Geometry check sheet. Reference: the model listing, model coordinates, mm. Round coordinates to 2 decimals unless told otherwise and drop trailing zeros. Order: outer loops, then holes, each group sorted by start corner. A loop starts at its lowest first (then second) coordinate and runs counter-clockwise, first axis right, second up. Notation, with made-up numbers: (28.5, 82) - (43.5, 82) arc R20 ccw to (43.5, 108) - close; hole circle Ø3 at (-2, 83). An arc over 180 degrees is marked (long way). Use a Markdown table: item, result. Add a question column.
(1) Section check A-A on x = 44. Record the boundary of the cut face in (y, z) (3 decimals), then the cut area to 4 significant figures.
(2) Gauge pin test, flat ends, axial feed: P1, Ø1, axis at x = 144.5, z = -1.5, coming from the +Y side; P2, Ø1.6, axis at y = -14, z = -1, coming from the -X side. Record the tip position at first contact, or that the pin passes through.
(3) Thickness scan on line 1 along X through (y, z) = (-157, -0.8); line 2 along X through (y, z) = (-180.6, -0.9); line 3 along Y through (x, z) = (216, -2.5). Record the ranges inside material, lowest first. Write a range as [from, to].
(4) Section check C-C on x = 115. Record the boundary of the cut face in (y, z) (3 decimals).
(5) Section check B-B on z = -0.55. Give the number of separate pieces and of enclosed holes in the cut face, then the cut area to 3 significant figures.
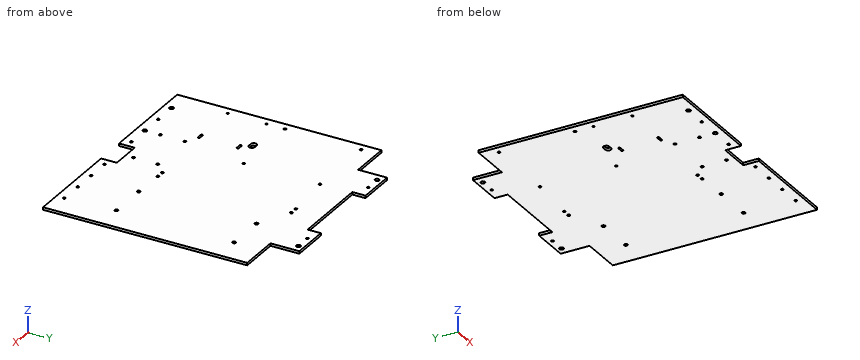
```python
from build123d import *

# Parameters (mm, degrees)
SKETCH1_W                    = 300
SKETCH1_H                    = 300
BOSS_EXTRUDE1_DEPTH          = 3.175
SKETCH2_W                    = 52
SKETCH2_H                    = 40
CUT_EXTRUDE1_DEPTH           = 10
M4_START                     = -3.175
M4_CLEARANCE_HOLE1_OUTLINE_R = 2.15
M4_CLEARANCE_HOLE1_DEPTH     = 3.175
M3_CLEARANCE_HOLE2_D         = 3.2
M2_5_CLEARANCE_HOLE1_D       = 2.7
M3_CLEARANCE_HOLE3_D         = 3.2
M3_CLEARANCE_HOLE4_D         = 3.2
CUT_EXTRUDE3_DEPTH           = 10
CUT_EXTRUDE4_DEPTH           = 10
SKETCH15_W                   = 40
SKETCH15_H                   = 20
CUT_EXTRUDE5_DEPTH           = 10
CUT_EXTRUDE6_START           = -10
CUT_EXTRUDE6_DEPTH           = 10
M3_CLEARANCE_HOLE5_D         = 3.4
M5_CLEARANCE_HOLE1_D         = 5.5
M3_CLEARANCE_HOLE7_D         = 3.4


# Read off the part's stored shape, not the designer's step: M4 Clearance Hole1
with BuildPart() as part:
    # Sketch1 → Boss-Extrude1 (new body)
    with BuildSketch(Plane(origin=(0, 0, 0), x_dir=(1, 0, 0), z_dir=(0, 0, -1))):
        with Locations((150, 150)):
            Rectangle(SKETCH1_W, SKETCH1_H)
    extrude(amount=BOSS_EXTRUDE1_DEPTH)

    # Sketch2 → Cut-Extrude1 (cut)
    with BuildSketch(Plane(origin=(0, 0, -3.175), x_dir=(1, 0, 0), z_dir=(0, 0, -1))):
        with Locations((26, 20)):
            Rectangle(SKETCH2_W, SKETCH2_H)
        with Locations((274, 20)):
            Rectangle(SKETCH2_W, SKETCH2_H)
    extrude(amount=-CUT_EXTRUDE1_DEPTH, mode=Mode.SUBTRACT)

    # M4 Clearance Hole1 outline → M4 Clearance Hole1 (cut)
    with BuildSketch(Plane.XY.offset(M4_START)):
        with Locations((266, -226)):
            Circle(M4_CLEARANCE_HOLE1_OUTLINE_R)
        with Locations((216, -76)):
            Circle(M4_CLEARANCE_HOLE1_OUTLINE_R)
        with Locations((216, -226)):
            Circle(M4_CLEARANCE_HOLE1_OUTLINE_R)
        with Locations((266, -76)):
            Circle(M4_CLEARANCE_HOLE1_OUTLINE_R)
    extrude(amount=M4_CLEARANCE_HOLE1_DEPTH, mode=Mode.SUBTRACT)

    # M3 Clearance Hole2 (through all)
    with Locations(Plane(origin=(0, 0, -3.175), x_dir=(-1, 0, 0), z_dir=(0, 0, -1))):
        with Locations((-102, -60), (-10, -157), (-102, -157), (-10, -60)):
            Hole(M3_CLEARANCE_HOLE2_D / 2)

    # M2.5 Clearance Hole1 (through all)
    with Locations(Plane(origin=(0, 0, -3.175), x_dir=(-1, 0, 0), z_dir=(0, 0, -1))):
        with Locations((-74, -180.6), (-10, -230), (-74, -230), (-10, -180.6), (-68, -230), (-68, -180.6)):
            Hole(M2_5_CLEARANCE_HOLE1_D / 2)

    # M3 Clearance Hole3 (through all)
    with Locations(Plane(origin=(0, 0, -3.175), x_dir=(-1, 0, 0), z_dir=(0, 0, -1))):
        with Locations((-30, -290), (-270, -290), (-240, -290), (-210, -290), (-180, -290), (-150, -290), (-120, -290), (-90, -290), (-60, -290)):
            Hole(M3_CLEARANCE_HOLE3_D / 2)

    # M3 Clearance Hole4 (through all)
    with Locations(Plane(origin=(0, 0, -3.175), x_dir=(-1, 0, 0), z_dir=(0, 0, -1))):
        with Locations((-82, -10), (-238, -10), (-150, -10), (-62, -10), (-218, -10)):
            Hole(M3_CLEARANCE_HOLE4_D / 2)

    # Sketch5 → Cut-Extrude3 (cut)
    with BuildSketch(Plane(origin=(0, 0, -3.175), x_dir=(-1, 0, 0), z_dir=(0, 0, -1))):
        Polygon((-248, 0), (-52, 0), (-52, -3.2), (-100, -3.2), (-100, -20), (-200, -20), (-200, -3.2), (-248, -3.2), align=None)
    extrude(amount=-CUT_EXTRUDE3_DEPTH, mode=Mode.SUBTRACT)

    # Sketch14 → Cut-Extrude4 (cut)
    with BuildSketch(Plane(origin=(0, 0, -3.175), x_dir=(-1, 0, 0), z_dir=(0, 0, -1))):
        with BuildLine():
            Line((-63, -165.2), (-59, -165.2))
            ThreePointArc((-59, -165.2), (-55.2, -169), (-59, -172.8))
            Line((-59, -172.8), (-63, -172.8))
            ThreePointArc((-63, -172.8), (-66.8, -169), (-63, -165.2))
        make_face()
    extrude(amount=-CUT_EXTRUDE4_DEPTH, mode=Mode.SUBTRACT)

    # Sketch15 → Cut-Extrude5 (cut)
    with BuildSketch(Plane(origin=(0, 0, -3.175), x_dir=(-1, 0, 0), z_dir=(0, 0, -1))):
        with Locations((-150, -290)):
            Rectangle(SKETCH15_W, SKETCH15_H)
    extrude(amount=-CUT_EXTRUDE5_DEPTH, mode=Mode.SUBTRACT)

    # Sketch16 → Cut-Extrude6 (cut)
    with BuildSketch(Plane(origin=(0, 0, -3.175), x_dir=(-1, 0, 0), z_dir=(0, 0, -1)).offset(CUT_EXTRUDE6_START)):
        with BuildLine():
            Line((-74, -179.25), (-68, -179.25))
            ThreePointArc((-68, -179.25), (-66.65, -180.6), (-68, -181.95))
            Line((-68, -181.95), (-74, -181.95))
            ThreePointArc((-74, -181.95), (-75.35, -180.6), (-74, -179.25))
        make_face()
        with BuildLine():
            Line((-74, -228.65), (-68, -228.65))
            ThreePointArc((-68, -228.65), (-66.65, -230), (-68, -231.35))
            Line((-68, -231.35), (-74, -231.35))
            ThreePointArc((-74, -231.35), (-75.35, -230), (-74, -228.65))
        make_face()
    extrude(amount=CUT_EXTRUDE6_DEPTH, mode=Mode.SUBTRACT)

    # M3 Clearance Hole5 (through all)
    with Locations(Plane(origin=(0, 0, -3.175), x_dir=(-1, 0, 0), z_dir=(0, 0, -1))):
        with Locations((-175, -55), (-165, -225), (-175, -225), (-165, -55)):
            Hole(M3_CLEARANCE_HOLE5_D / 2)

    # M5 Clearance Hole1 (through all)
    with Locations(Plane(origin=(0, 0, -3.175), x_dir=(-1, 0, 0), z_dir=(0, 0, -1))):
        with Locations((-62, -10), (-90, -290), (-30, -290), (-238, -10)):
            Hole(M5_CLEARANCE_HOLE1_D / 2)

    # M3 Clearance Hole7 (through all)
    with Locations(Plane(origin=(0, 0, -3.175), x_dir=(-1, 0, 0), z_dir=(0, 0, -1))):
        with Locations((-150.5, -239), (-90, -270), (-150.5, -270), (-90, -239)):
            Hole(M3_CLEARANCE_HOLE7_D / 2)


solid = part.part
```
Check sheet entries:
| question | item | result |
|---|---|---|
| 1 | outline | (-300, -3.175) - (-40, -3.175) - (-40, 0) - (-300, 0) - close |
| 1 | area | 825.5 mm2 |
| 2 | P1 | stops at y = -20 |
| 2 | P2 | stops at x = 52 |
| 3 | line 1 | x = [0, 8.4], [11.6, 100.4], [103.6, 300] |
| 3 | line 2 | x = [0, 8.65], [11.35, 66.65], [75.35, 300] |
| 3 | line 3 | y = [-300, -228.15], [-223.85, -78.15], [-73.85, -3.2] |
| 4 | outline | (-300, -3.175) - (-20, -3.175) - (-20, 0) - (-300, 0) - close |
| 5 | separate pieces | 1 |
| 5 | enclosed holes | 33 |
| 5 | area | 82,300 mm2 |
